```python
from build123d import *

# Parameters (mm, degrees)
SKETCH_W          = 60
SKETCH_H          = 40
SKETCH_W_2        = 50
SKETCH_H_2        = 30
PAD_DEPTH         = 5
SKETCH001_W       = 5
SKETCH001_H       = 5
PAD001_DEPTH      = 40
SKETCH002_W       = 60
SKETCH002_H       = 40
SKETCH002_W_2     = 50
SKETCH002_H_2     = 30
PAD002_DEPTH      = 5
SKETCH003_W       = 10
SKETCH003_H       = 5
PAD003_DEPTH      = 30
SKETCH004_W       = 5
SKETCH004_H       = 8
PAD004_DEPTH      = 10
SKETCH005_R       = 12.5
PAD005_DEPTH      = 10
PAD005_DEPTH_BACK = 10
SKETCH006_R       = 10.5
POCKET_DEPTH      = 42.501
SKETCH007_W       = 5
SKETCH007_H       = 8
PAD006_DEPTH      = 10
SKETCH008_R       = 12.5
PAD007_DEPTH      = 10
PAD007_DEPTH_BACK = 10
SKETCH009_R       = 10.5
POCKET001_DEPTH   = 42.570779
SKETCH010_W       = 10
SKETCH010_H       = 5
PAD008_DEPTH      = 40
SKETCH011_R       = 12.5
PAD009_DEPTH      = 12
PAD009_DEPTH_BACK = 5
SKETCH012_R       = 10.5
POCKET002_DEPTH   = 17.001
FILLET_R          = 2
FILLET001_R       = 2
FILLET002_R       = 2
FILLET003_R       = 2
FILLET004_R       = 2
FILLET005_R       = 2
FILLET006_R       = 2
FILLET007_R       = 2


with BuildPart() as part:
    # Sketch → Pad (new body)
    with BuildSketch(Plane.XZ):
        with Locations((0, 20)):
            Rectangle(SKETCH_W, SKETCH_H)
        with Locations((0, 20)):
            Rectangle(SKETCH_W_2, SKETCH_H_2, mode=Mode.SUBTRACT)
    extrude(amount=PAD_DEPTH)

    # Sketch001 (on Face10 of Pad) → Pad001 (join)
    with BuildSketch(Plane.XZ.offset(5)):
        with Locations((-27.5, 37.5)):
            Rectangle(SKETCH001_W, SKETCH001_H)
        with Locations((27.5, 37.5)):
            Rectangle(SKETCH001_W, SKETCH001_H)
        with Locations((27.5, 2.5)):
            Rectangle(SKETCH001_W, SKETCH001_H)
        with Locations((-27.5, 2.5)):
            Rectangle(SKETCH001_W, SKETCH001_H)
    extrude(amount=PAD001_DEPTH)

    # Sketch002 (on Face10 of Pad001) → Pad002 (join)
    with BuildSketch(Plane.XZ.offset(45)):
        with Locations((0, 20)):
            Rectangle(SKETCH002_W, SKETCH002_H)
        with Locations((0, 20)):
            Rectangle(SKETCH002_W_2, SKETCH002_H_2, mode=Mode.SUBTRACT)
    extrude(amount=PAD002_DEPTH)

    # Sketch003 (on Face26 of Pad002) → Pad003 (join)
    with BuildSketch(Plane(origin=(0, 0, 5), x_dir=(-1, 0, 0), z_dir=(0, 0, 1))):
        with Locations((0, 47.5)):
            Rectangle(SKETCH003_W, SKETCH003_H)
        with Locations((0, 2.5)):
            Rectangle(SKETCH003_W, SKETCH003_H)
    extrude(amount=PAD003_DEPTH)

    # Sketch004 (on Face36 of Pad003) → Pad004 (join)
    with BuildSketch(Plane.XZ.offset(50)):
        with Locations((0, 20)):
            Rectangle(SKETCH004_W, SKETCH004_H)
    extrude(amount=PAD004_DEPTH)

    # Sketch005 (on Face19 of Pad004) → Pad005 (join, two sides)
    with BuildSketch(Plane(origin=(-2.5, 0, 0), x_dir=(0, 0, -1), z_dir=(-1, 0, 0))) as pad005_sk:
        with Locations((-20, 69)):
            Circle(SKETCH005_R)
    extrude(amount=PAD005_DEPTH)
    extrude(pad005_sk.sketch, amount=-PAD005_DEPTH_BACK)

    # Sketch006 (on Face43 of Pad005) → Pocket (cut, through all)
    with BuildSketch(Plane(origin=(-12.5, 0, 0), x_dir=(0, 0, -1), z_dir=(-1, 0, 0))):
        with Locations((-20, 69)):
            Circle(SKETCH006_R)
        with Locations((-20, 69)):
            Circle(SKETCH006_R)
    extrude(amount=-POCKET_DEPTH, mode=Mode.SUBTRACT)

    # Sketch007 (on Face26 of Pocket) → Pad006 (join)
    with BuildSketch(Plane(origin=(0, 0, 0), x_dir=(1, 0, 0), z_dir=(0, 1, 0))):
        with Locations((-0.069779, -20)):
            Rectangle(SKETCH007_W, SKETCH007_H)
    extrude(amount=PAD006_DEPTH)

    # Sketch008 (on Face42 of Pad006) → Pad007 (join, two sides)
    with BuildSketch(Plane(origin=(-2.569779, 0, 0), x_dir=(0, 0, -1), z_dir=(-1, 0, 0))) as pad007_sk:
        with Locations((-20, -19)):
            Circle(SKETCH008_R)
    extrude(amount=PAD007_DEPTH)
    extrude(pad007_sk.sketch, amount=-PAD007_DEPTH_BACK)

    # Sketch009 (on Face51 of Pad007) → Pocket001 (cut, through all)
    with BuildSketch(Plane(origin=(-12.569779, 0, 0), x_dir=(0, 0, -1), z_dir=(-1, 0, 0))):
        with Locations((-20, -19)):
            Circle(SKETCH009_R)
    extrude(amount=-POCKET001_DEPTH, mode=Mode.SUBTRACT)

    # Sketch010 (on Face2 of Pocket001) → Pad008 (join)
    with BuildSketch(Plane(origin=(0, -45, 0), x_dir=(1, 0, 0), z_dir=(0, 1, 0))):
        with Locations((0, -2.5)):
            Rectangle(SKETCH010_W, SKETCH010_H)
    extrude(amount=PAD008_DEPTH)

    # Sketch011 (on Face22 of Pad008) → Pad009 (join, two sides)
    with BuildSketch(Plane(origin=(0, 0, 5), x_dir=(-1, 0, 0), z_dir=(0, 0, 1))) as pad009_sk:
        with Locations((0, 25)):
            Circle(SKETCH011_R)
    extrude(amount=PAD009_DEPTH)
    extrude(pad009_sk.sketch, amount=-PAD009_DEPTH_BACK)

    # Sketch012 (on Face44 of Pad009) → Pocket002 (cut, through all)
    with BuildSketch(Plane(origin=(0, 0, 17), x_dir=(-1, 0, 0), z_dir=(0, 0, 1))):
        with Locations((0, 25)):
            Circle(SKETCH012_R)
    extrude(amount=-POCKET002_DEPTH, mode=Mode.SUBTRACT)

    # Fillet
    fillet_edges = [part.edges().sort_by_distance(p)[0] for p in [
        (-30, -25, 40),
    ]]
    fillet(fillet_edges, radius=FILLET_R)

    # Fillet001
    fillet001_edges = [part.edges().sort_by_distance(p)[0] for p in [
        (-30, -25, 0),
    ]]
    fillet(fillet001_edges, radius=FILLET001_R)

    # Fillet002
    fillet002_edges = [part.edges().sort_by_distance(p)[0] for p in [
        (30, -25, 40),
    ]]
    fillet(fillet002_edges, radius=FILLET002_R)

    # Fillet003
    fillet003_edges = [part.edges().sort_by_distance(p)[0] for p in [
        (30, -25, 0),
    ]]
    fillet(fillet003_edges, radius=FILLET003_R)

    # Fillet004
    fillet004_edges = [part.edges().sort_by_distance(p)[0] for p in [
        (-2.5, -53.57864, 24),
    ]]
    fillet(fillet004_edges, radius=FILLET004_R)

    # Fillet005
    fillet005_edges = [part.edges().sort_by_distance(p)[0] for p in [
        (-2.5, -53.57864, 16),
    ]]
    fillet(fillet005_edges, radius=FILLET005_R)

    # Fillet006
    fillet006_edges = [part.edges().sort_by_distance(p)[0] for p in [
        (-2.569779, 3.57864, 24),
    ]]
    fillet(fillet006_edges, radius=FILLET006_R)

    # Fillet007
    fillet007_edges = [part.edges().sort_by_distance(p)[0] for p in [
        (-2.569779, 3.57864, 16),
    ]]
    fillet(fillet007_edges, radius=FILLET007_R)


solid = part.part
```
Verification items for the finished model (mm, model axes). A direction names the side the tool comes from. Give positions to 0.01 mm unless a question says otherwise; leave off trailing zeros. Order: outer loops, then holes, each group sorted by start corner. A loop starts at its lowest first (then second) coordinate and runs counter-clockwise, first axis right, second up. Notation, with made-up numbers: M 61.5,8.5 L 106.5,8.5 A20 cw 106.5,13.5 Z; hole C -28,38 d10. An arc over 180 degrees is marked long. Return JSON: item names as keys, results as strings. Group by question number.
1) Section check A-A on y = -69. Record the cut outline in (x, z), and give its area (3 significant figures).
2) Scan lines: line 1 (X direction, y = -25, z = 4.25); line 2 (Y direction, x = 0, z = 7); line 3 (Z direction, x = 24.5, y = -49). Record each from-to range of solid material in increasing order.
3) Access from +Z, -Z, +X, -X, +Y, -Y to the whole of each face (thin tool, end or side, straight path). Record for faces 1 (the face through (25, -25, 37)), 2 (the face through (-25, -2, 20)), 3 (the face through (5, -2, 20)).
4) Go/stop test with flat-tipped pins: pin 1 Ø1 at (x, y) = (-2, 6) entering from -Z; pin 2 Ø1 at (x, y) = (-5.5, -59) entering from +Z; pin 3 Ø10 at (x, z) = (11.5, 12.5) entering from -Y. Record where each tip stops, or that it passes through.
5) Mould release check, pull along X, two halves, no side actions. Record for faces 4 (the face through (-30, -25, 36)), 5 (the face through (-5, -9, 3)), 6 (the face through (0, -14, 0)): pulls with the +X half, pulls with the -X half, needs draft (parallel to the pull), parting line crosses it, or undercut.
6) Section check B-B on z = 3.5. Record the cut outline in (x, y).
7) Section check D-D on y = 5. Record the cut outline in (x, z), and give its area (3 significant figures).
8) Section check C-C on x = 16. Record the cut outline in (y, z).
Answer block:
{
 "1": {"outline": "M -12.5,7.5 L 7.5,7.5 L 7.5,9.5 L -12.5,9.5 Z; M -12.5,30.5 L 7.5,30.5 L 7.5,32.5 L -12.5,32.5 Z", "area": "80.0 mm^2"},
 "2": {"line 1": "x = -30 to -25, -12.5 to -10.5, 10.5 to 12.5, 25 to 30", "line 2": "y = -50 to -45, -37.5 to -35.5, -14.5 to -12.5, -5 to 0", "line 3": "z = 0 to 5, 35 to 40"},
 "3": {"face 1": "+Z, -Z", "face 2": "+Y, -Y", "face 3": "none"},
 "4": {"pin 1": "stops at z = 16.23", "pin 2": "stops at z = 28.12", "pin 3": "stops at y = -80.66"},
 "5": {"face 4": "pulls with the -X half", "face 5": "undercut", "face 6": "needs draft"},
 "6": {"outline": "M -30,-50 L 30,-50 L 30,0 L -30,0 Z; hole M -25,-45 L -5,-45 L -5,-36.46 A12.5 cw -5,-13.54 L -5,-5 L -25,-5 Z; hole C 0,-25 d21; hole M 5,-45 L 25,-45 L 25,-5 L 5,-5 L 5,-13.54 A12.5 cw 5,-36.46 Z"},
 "7": {"outline": "M -2.57,18 A2 ccw -0.57,16 L 2.43,16 L 2.43,24 L -0.57,24 A2 ccw -2.57,22 Z", "area": "38.3 mm^2"},
 "8": {"outline": "M -50,0 L -45,0 L -45,5 L -50,5 Z; M -50,35 L -45,35 L -45,40 L -50,40 Z; M -5,0 L 0,0 L 0,5 L -5,5 Z; M -5,35 L 0,35 L 0,40 L -5,40 Z"}
}
